Autodesk Inventor part; units mm, degrees
ref_plane "YZ Plane" through (0, 0, 0) normal (1, 0, 0) x (0, 1, 0)
ref_plane "XZ Plane" through (0, 0, 0) normal (0, 1, 0) x (-1, 0, 0)
ref_plane "XY Plane" through (0, 0, 0) normal (0, 0, 1) x (1, 0, 0)
sketch "Sketch1" plane through (0, 0, 0) normal (0, 1, 0) x (-1, 0, 0)
  circle A0 centre (0, 0) radius 1.5
  circle A1 centre (0, 0) radius 6
  line L0 (13.4781, 0) -> (13.4781, -4)
  line L1 (13.4781, 0) -> (13.4781, 4)
  line L2 (13.4781, 4) -> (0, 6)
  line L3 (13.4781, -4) -> (0, -6)
  dimension "d0" = 3
  dimension "d1" = 12
  dimension "d2" = 4
extrude "Extrusion1" add sketch "Sketch1" along normal mid plane 4.5 contours L2 A1 L3 | L2 L1 L0 L3 A1
sketch "Sketch2" plane through (-13.4781, -2.25, -4) normal (-1, 0, 0) x (0, 0, 1)
  line L0 (2.5, 4.5) -> (2.5, 0)
  line L1 (8, 0) -> (0, 0)
  line L2 (8, 4.5) -> (8, 0)
  line L3 (0, 4.5) -> (8, 4.5)
  line L4 (0, 0) -> (0, 4.5)
  circle A0 centre (4, 2.25) radius 2
  dimension "d5" = 4
extrude "Extrusion2" add sketch "Sketch2" along normal blind 60 contours A0 L0 | L0 A0
fillet "Fillet1" [suppressed]
sketch "Sketch4" plane through (0, 0, 0) normal (0, 1, 0) x (-1, 0, 0)
  line L0 (13.4781, 4) -> (0, 6)
  arc A0 (0, 6) -> (0, -6) centre (0, 0) ccw
  line L1 (0, -6) -> (13.4781, -4)
  line L2 (13.4781, -4) -> (13.4781, 4)
  circle A1 centre (0, 0) radius 1.5
  line L3 (13.4781, 4) -> (13.4781, -4)
  line L4 (13.4781, 0) -> (17.6846, 0)
  line L5 (17.6846, 0) -> (17.6846, 0.0214)
  line L6 (17.6846, -11.5062) -> (15.4451, -11.5062)
  line L7 (15.4451, -11.5062) -> (15.4451, -13.5813)
  line L8 (15.4451, -13.5813) -> (14.6622, -13.5813)
  line L9 (13.4781, -4) -> (13.4781, -5.198)
  line L10 (13.4781, -5.198) -> (14.6622, -13.5813)
  line L11 (17.6846, -11.5062) -> (17.6846, -10.8233)
  line L12 (17.6846, -10.8233) -> (15.4853, -10.8233)
  line L13 (15.4853, -10.8233) -> (15.0537, -7.0356)
  line L14 (15.0537, -7.0356) -> (15.0537, 0)
  dimension "d13" = 11.5062
revolve "Revolution1" add sketch "Sketch4" angle 360 about axis through (-13.4781, 0, 0) along (-1, 0, 0) contours L4 L14 L13 L12 L11 L6 L7 L8 L10 L9 L2
properties part number "100MMshockLower"
Geometry: final body of the model. Coordinates: model frame, mm. A direction names the side the tool comes from. Give positions to 0.01 mm unless a question says otherwise; leave off trailing zeros. Loops run counter-clockwise (first coordinate to the right, second up) from the corner with the lowest first, then second, coordinate; pieces in that order, holes last. Notation, with made-up numbers: (69.5, -35) - (75.5, -35) arc R10 ccw to (75.5, -27) - close; hole circle Ø8 at (-18, -29). An arc over 180 degrees is marked (long way). Answer as CSV lines item,"result". Start each with the question number.
(1) Section query B-B (y = 0). Output: boundary loops of the cut face in (x, z).
(2) Reachability of faces 1 (the face through (-15.054, 1, 2)), 2 (the face through (-4, -2.25, 0)), 3 (the face through (-6.833, -0.031, 4.986)), 4 (the face through (-4, 2.25, 0)) from +Z, -Z, +X, -X, +Y, -Y: full face, straight path, thin tool, end or side. Return the list, or none.
(3) Ray query, line 1 along Y through (x, z) = (-16.65, 0); line 2 along Z through (x, y) = (0, -0.05); line 3 along Y through (x, z) = (-13, -0.75). Return the intervals inside material, ascending. Write a range as [from, to].
(4) Mould query, pull axis X, two halves, no side actions, for faces 5 (the face through (6, 0, 0)), 6 (the face through (-16.549, -11.233, 2.494)), 7 (the face through (-6.833, -0.031, -4.986)). Classes: +X half, -X half, draft (parallel to the pull), parting line (faces both ways), or undercut.
(5) Section query C-C (x = -67). Output: boundary loops of the cut face in (y, z), and give its area (3 significant figures).
(6) Section query A-A (z = 0). Output: boundary loops of the cut face in (x, y), and give its area (3 significant figures).
(7) Pin query (flat end, axial travel): P1, Ø4, axis at x = 0, z = 0, coming from the -Y side; P2, Ø9.5, axis at x = -3, z = 0.5, coming from the +Y side; P3, Ø5, axis at x = -36, z = 2, coming from the -Y side. Return the tip coordinate at first contact, or that it passes through.
Worked answers:
1,outline,"(-73.48, -2) - (-15.05, -2) - (-15.05, -7.04) - (-15.49, -10.82) - (-17.68, -10.82) - (-17.68, -11.51) - (-15.45, -11.51) - (-15.45, -13.58) - (-14.66, -13.58) - (-13.48, -5.2) - (-13.48, -4) - (0, -6) arc R6 ccw to (0, 6) - (-13.48, 4) - (-13.48, 5.2) - (-14.66, 13.58) - (-15.45, 13.58) - (-15.45, 11.51) - (-17.68, 11.51) - (-17.68, 10.82) - (-15.49, 10.82) - (-15.05, 7.04) - (-15.05, 2) - (-73.48, 2) - close; hole circle Ø3 at (0, 0)"
2,face 1,"-X"
2,face 2,"+Z, -Z, +X, -Y"
2,face 3,"+Z, +Y, -Y"
2,face 4,"+Z, -Z, +X, +Y"
3,line 1,"y = [-11.51, -10.82], [-2, 2], [10.82, 11.51]"
3,line 2,"z = [-6, -1.5], [1.5, 6]"
3,line 3,"y = [-2.25, 2.25]"
4,face 5,"+X half"
4,face 6,"draft"
4,face 7,"undercut"
5,outline,"circle Ø4 at (0, 0)"
5,area,"12.6 mm^2"
6,outline,"(-73.48, -2) - (-15.05, -2) - (-15.05, -7.04) - (-15.49, -10.82) - (-17.68, -10.82) - (-17.68, -11.51) - (-15.45, -11.51) - (-15.45, -13.58) - (-14.66, -13.58) - (-13.48, -5.2) - (-13.48, -2.25) - (-1.5, -2.25) - (-1.5, 2.25) - (-13.48, 2.25) - (-13.48, 5.2) - (-14.66, 13.58) - (-15.45, 13.58) - (-15.45, 11.51) - (-17.68, 11.51) - (-17.68, 10.82) - (-15.49, 10.82) - (-15.05, 7.04) - (-15.05, 2) - (-73.48, 2) - close; (1.5, -2.25) - (6, -2.25) - (6, 2.25) - (1.5, 2.25) - close"
6,area,"348 mm^2"
7,P1,"stops at y = -2.25"
7,P2,"stops at y = 2.25"
7,P3,"stops at y = -2"
